from build123d import *

# Parameters (mm, degrees)
F1_DEPTH = 4
F3_DEPTH = 5
F4_W     = 20
F4_H     = 44.5
F5_DEPTH = 7
F6_W     = 25
F6_H     = 5
F7_DEPTH = 13


with BuildPart() as f1:
    # F0 (on Top) → F1 (new body)
    with BuildSketch(Plane.XY):
        with BuildLine():
            ThreePointArc((25, 15), (22.071068, 22.071068), (15, 25))
            Line((15, 25), (-15, 25))
            ThreePointArc((-15, 25), (-22.071068, 22.071068), (-25, 15))
            Line((-25, 15), (-25, -15))
            ThreePointArc((-25, -15), (-22.071068, -22.071068), (-15, -25))
            Line((-15, -25), (15, -25))
            ThreePointArc((15, -25), (22.071068, -22.071068), (25, -15))
            Line((25, -15), (25, 15))
        make_face()
    extrude(amount=F1_DEPTH)

    # F2 (on face) → F3 (join)
    with BuildSketch(Plane.XY.offset(4)):
        with BuildLine():
            ThreePointArc((22.25, 14.75), (20.053301, 20.053301), (14.75, 22.25))
            Line((14.75, 22.25), (-14.75, 22.25))
            ThreePointArc((-14.75, 22.25), (-20.053301, 20.053301), (-22.25, 14.75))
            Line((-22.25, 14.75), (-22.25, -14.75))
            ThreePointArc((-22.25, -14.75), (-20.053301, -20.053301), (-14.75, -22.25))
            Line((-14.75, -22.25), (14.75, -22.25))
            ThreePointArc((14.75, -22.25), (20.053301, -20.053301), (22.25, -14.75))
            Line((22.25, -14.75), (22.25, 14.75))
        make_face()
    extrude(amount=F3_DEPTH)

    # F4 (on face) → F5 (cut)
    with BuildSketch(Plane.XY.offset(9)):
        Rectangle(F4_W, F4_H)
    extrude(amount=-F5_DEPTH, mode=Mode.SUBTRACT)

    # F6 (on face) → F7 (cut)
    with BuildSketch(Plane.YZ.offset(22.25)):
        with Locations((-4.5, 6.5)):
            Rectangle(F6_W, F6_H)
    extrude(amount=-F7_DEPTH, mode=Mode.SUBTRACT)


solid = f1.part
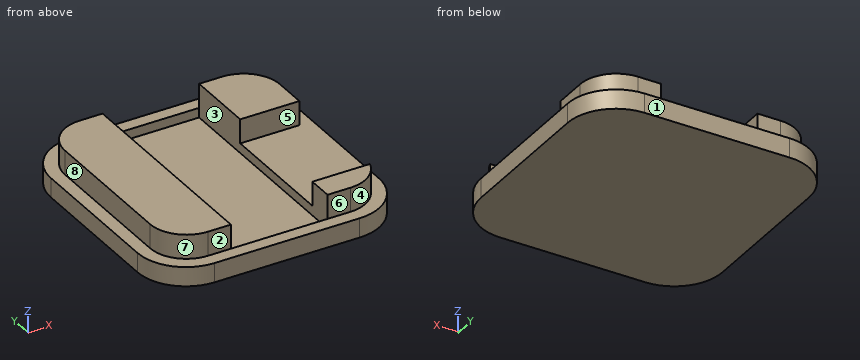
Source: CAD feature listing. Evaluate the final solid. Frame: model axes, mm. Face numbers are marked on the shaded views. A direction names the side the tool comes from. Coordinates: 2 decimals unless noted, no trailing zeros. Order: outer loops, then holes, each group sorted by start corner. A loop starts at its lowest first (then second) coordinate and runs counter-clockwise, first axis right, second up.
Item 1: Set-up query: the marked faces 4, 5, 6, 7 and 8. Return all of +Z, -Z, +X, -X, +Y, -Y with unobstructed straight access to the full face (end or side cutting, diameter ignored); none if empty.
Output values:
face 4: +Z, +X, -Y
face 5: +Z, +X
face 6: +Z, +X, -X, -Y
face 7: +Z, -X, -Y
face 8: +Z, -X, +Y, -Y
Item 2: Cut plane C-C (y = -4.5). Return loops of the section in (x, z).
Output values:
outline: (-25, 0) - (25, 0) - (25, 4) - (10, 4) - (10, 2) - (-10, 2) - (-10, 9) - (-22.25, 9) - (-22.25, 4) - (-25, 4) - close
Item 3: Cut plane D-D (x = -16.5). Return loops of the section in (y, z), plus the area to 3 significant figures.
Output values:
outline: (-24.89, 0) - (24.89, 0) - (24.89, 4) - (22.04, 4) - (22.04, 9) - (-22.04, 9) - (-22.04, 4) - (-24.89, 4) - close
area: 420 mm2
Item 4: Pull-direction query (Y, two-part tool) for the marked faces 1, 2 and 3; classes: pulls with the +Y half, pulls with the -Y half, needs draft (parallel to the pull), parting line crosses it, or undercut.
Output values:
face 1: pulls with the +Y half
face 2: pulls with the -Y half
face 3: undercut
Item 5: First-contact query: P1, Ø5, axis at x = 11.5, z = 7, coming from the -Y side; P2, Ø5, axis at x = -13, z = 7, coming from the +Y side; P3, Ø6, axis at x = 2, y = 5, coming from the +Z side; P4, Ø2, axis at x = 2.5, y = -3.5, coming from the -Z side. Flat tips, straight axial feed; report the tip coordinate or a pass-through.
Output values:
P1: stops at y = -22.25
P2: stops at y = 22.25
P3: stops at z = 2
P4: stops at z = 0
Item 6: Cut plane B-B (x = -1). Return loops of the section in (y, z), plus the area to 3 significant figures.
Output values:
outline: (-25, 0) - (25, 0) - (25, 4) - (22.25, 4) - (22.25, 2) - (-22.25, 2) - (-22.25, 4) - (-25, 4) - close
area: 111 mm2
Item 7: Material intervals for line 1 (X direction, y = 9, z = 8.25); line 2 (Y direction, x = 6.5, z = 3.5); line 3 (X direction, y = 7, z = 2.75), sorted ascending.
Output values:
line 1: x = -22.25 to -10, 10 to 22.25
line 2: y = -25 to -22.25, 22.25 to 25
line 3: x = -25 to -10, 10 to 25
Item 8: Cut plane A-A (z = 5.75). Return loops of the section in (x, y), plus the area to 3 significant figures.
Output values:
outline: (-22.25, -14.75) arc R7.5 ccw to (-14.75, -22.25) - (-10, -22.25) - (-10, 22.25) - (-14.75, 22.25) arc R7.5 ccw to (-22.25, 14.75) - close; (10, -22.25) - (14.75, -22.25) arc R7.5 ccw to (21.9, -17) - (10, -17) - close; (10, 8) - (22.25, 8) - (22.25, 14.75) arc R7.5 ccw to (14.75, 22.25) - (10, 22.25) - close
area: 736 mm2
